Work out the finished part from the listing and answer in its coordinate system (mm). Coordinates: 2 decimals unless noted, no trailing zeros. Order: outer loops, then holes, each group sorted by start corner. A loop starts at its lowest first (then second) coordinate and runs counter-clockwise, first axis right, second up. Notation, with made-up numbers: M 17,35.5 L 22,35.5 A29 ccw 22,64.5 Z; hole C 11,1 d3. An arc over 180 degrees is marked long. Write item = value, one per line. Start each with the question number.
Q1. Find section B-B on x = -84. Give the vertices of the cut face in (y, z).
Q2. Find section A-A on z = 12.75. Give the vertices of the cut face in (x, y).
Q3. Straight lines are drawn through the part: line 1 along X through (y, z) = (-14, 6.5); line 2 along X through (y, z) = (-4, 12); line 3 along Y through (x, z) = (-20.5, 5.5). For each, find the intervals that lie inside material, in ascending order.
Q4. Find section C-C on z = 3.5. Give the vertices of the cut face in (x, y), and give its area (3 significant figures).
Q5. Each of these flat-tipped pins is pushed along its axis until it touches: P1, Ø5, axis at x = -115, z = 5.5, coming from the -Y side; P2, Ø8, axis at x = -94.5, z = 7.5, coming from the +Y side; P3, Ø4, axis at y = 27, z = 7.5, coming from the +X side. Where does it stop, or does it pass through?
```python
from build123d import *

# Parameters (mm, degrees)
F0_R     = 17.5
F0_W     = 10
F0_H     = 30
F0_W_2   = 8
F0_H_2   = 15
F1_DEPTH = 15
F2_R     = 5


with BuildPart() as f1:
    # F0 (on Top) → F1 (new body)
    with BuildSketch(Plane.XY):
        with BuildLine():
            Line((0, 30.9548118476), (-155, 30.9548118476))
            Line((-155, 30.9548118476), (-155, 0))
            Line((-155, 0), (-145, 0))
            Line((-145, 0), (-130.978256464, 0))
            Line((-130.978256464, 0), (-122.978256464, 0))
            Line((-122.978256464, 0), (-111.2298741937, 0))
            Line((-111.2298741937, 0), (-97.2298741937, 0))
            Line((-97.2298741937, 0), (0, 0))
            ThreePointArc((0, 0), (66.3918764312, 15.4774059238), (0, 30.9548118476))
        make_face()
        with Locations((31.3918764312, 15.4774059238)):
            Circle(F0_R, mode=Mode.SUBTRACT)
        with Locations((-150, -15)):
            Rectangle(F0_W, F0_H)
        with Locations((-126.978256464, -7.5)):
            Rectangle(F0_W_2, F0_H_2)
        Polygon((-104.2298741937, -14.3756624311), (-97.2298741937, 0), (-111.2298741937, 0), align=None)
    extrude(amount=F1_DEPTH)

    # F2
    f2_edges = [f1.edges().sort_by_distance(p)[0] for p in [
        (-150, -30, 15),
        (-155, 0.477406, 15),
        (-137.989128, 0, 15),
        (-130.978256, -7.5, 15),
        (-107.729874, -7.187831, 15),
        (-117.104065, 0, 15),
        (-48.614937, 0, 15),
        (-77.5, 30.954812, 15),
        (66.391876, 15.477406, 15),
        (13.891876, 15.477406, 15),
    ]]
    fillet(f2_edges, radius=F2_R)


solid = f1.part
```
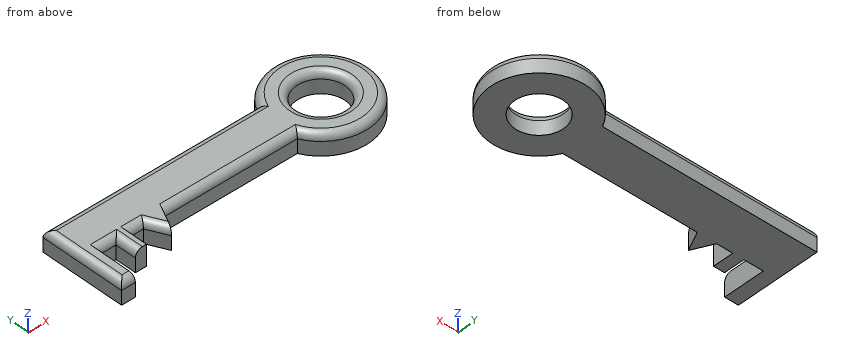
Findings below:
q1.outline = M 0,0 L 30.95,0 L 30.95,10 A5 ccw 25.95,15 L 5,15 A5 ccw 0,10 Z
q2.outline = M -154.18,-29.18 L -145,-29.18 L -145,0.82 L -130.15,0.82 L -130.15,-15 L -122.98,-15 L -122.98,0.82 L -110.71,0.82 L -103.77,-13.43 L -96.83,0.82 L 0.52,0.82 A34.18 ccw long 0.52,30.13 L -154.18,30.13 Z; hole C 31.39,15.48 d36.65
q3.line_1 = -155 to -145, -130.98 to -122.98, -104.41 to -104.05, 12.52 to 50.26
q3.line_2 = -154.58 to -145, -130.56 to -122.98, -108.82 to -99.18, 2.82 to 59.97
q3.line_3 = 0 to 30.95
q4.outline = M -155,-30 L -145,-30 L -145,0 L -130.98,0 L -130.98,-15 L -122.98,-15 L -122.98,0 L -111.23,0 L -104.23,-14.38 L -97.23,0 L 0,0 A35 ccw long 0,30.95 L -155,30.95 Z; hole C 31.39,15.48 d35
q4.area = 8,130 mm^2
q5.P1 = 0
q5.P2 = 30.95
q5.P3 = 65.07
